Autodesk Inventor part; units mm, degrees
ref_plane "Work Plane1" through (0, 0, 0) normal (0, 0, 1) x (1, 0, 0)
ref_plane "YZ Plane" through (0, 0, 0) normal (1, 0, 0) x (0, 1, 0)
ref_plane "XZ Plane" through (0, 0, 0) normal (0, 1, 0) x (-1, 0, 0)
ref_plane "Work Plane1" through (0, 0, 0) normal (0, 0, 1) x (1, 0, 0)
sketch "Sketch1" plane through (0, 0, 0) normal (0, 0, 1) x (1, 0, 0)
  arc A0 (-0.0454, -1100) -> (0.0454, -1099.9979) centre (-0.0454, -1098) ccw
  line L0 (0.0454, -1099.9979) -> (975.903, -1055.6408)
  arc A1 (975.903, -1055.6408) -> (1100, -925.7749) centre (970, -925.7749) ccw
  line L1 (1100, -174.2251) -> (1100, -925.7749)
  arc A2 (1100, -174.2251) -> (975.903, -44.3592) centre (970, -174.2251) ccw
  line L2 (0.0454, -0.0021) -> (975.903, -44.3592)
  arc A3 (0.0454, -0.0021) -> (-0.0454, 0) centre (-0.0454, -2) ccw
  line L3 (-0.0454, 0) -> (-470, 0)
  arc A4 (-470, 0) -> (-600, -130) centre (-470, -130) ccw
  line L4 (-600, -970) -> (-600, -130)
  arc A5 (-600, -970) -> (-470, -1100) centre (-470, -970) ccw
  line L5 (-0.0454, -1100) -> (-470, -1100)
  point P0 (0, 0)
extrude "Plate1" add sketch "Sketch1" against normal blind 1.5
equation "\"d0\" = Thickness"
equation "\"BendRadius\" = Thickness"
equation "\"BendReliefWidth\" = Thickness"
equation "\"BendReliefDepth\" = 0.5 * Thickness"
equation "\"CornerReliefSize\" = 4 * Thickness"
equation "\"MinimumRemnant\" = 2 * Thickness"
equation "\"TransitionRadius\" = BendRadius"
equation "\"JacobiRadiusSize\" = BendRadius"
equation "\"GapSize\" = Thickness"
properties part number "CARCASA_ALUM_4"
Part model, mm, in its own coordinate system. Round coordinates to 2 decimals unless told otherwise and drop trailing zeros. Loops run counter-clockwise (first coordinate to the right, second up) from the corner with the lowest first, then second, coordinate; pieces in that order, holes last. Notation, with made-up numbers: (54.5, 5.25) -> (63.5, 5.25) arc R23 ccw to (63.5, 31.25) -> close; hole circle Ø11 at (51.5, 35). An arc over 180 degrees is marked (long way). Use a Markdown table: item, result.
1) Cut at C-C, the plane y = -90. List the corners of the cut face in (x, z).
The answers:
| item | result |
|---|---|
| outline | (-593.69, -1.5) -> (1069.03, -1.5) -> (1069.03, 0) -> (-593.69, 0) -> close |
2) Cut at A-A, the plane z = -0.3. List the corners of the cut face in (x, y).
The answers:
| item | result |
|---|---|
| outline | (-600, -970) arc R130 ccw to (-470, -1100) -> (-0.05, -1100) arc R1.93 ccw to (0.05, -1100) -> (975.9, -1055.64) arc R130 ccw to (1100, -925.77) -> (1100, -174.23) arc R130 ccw to (975.9, -44.36) -> (0.05, 0) arc R2.08 ccw to (-0.05, 0) -> (-470, 0) arc R130 ccw to (-600, -130) -> close |
3) Cut at B-B, the plane x = 270.5. List the corners of the cut face in (y, z).
The answers:
| item | result |
|---|---|
| outline | (-1087.7, -1.5) -> (-12.3, -1.5) -> (-12.3, 0) -> (-1087.7, 0) -> close |
4) Probe line 1 (X direction, y = -955, z = -1.3); line 2 (Y direction, x = 97, z = -1); line 3 (Y direction, x = 915.5, z = -0.7). List the from-to ranges inside material, lowest first. Write a range as [from, to].
The answers:
| item | result |
|---|---|
| line 1 | x = [-600, 1096.67] |
| line 2 | y = [-1095.59, -4.41] |
| line 3 | y = [-1058.39, -41.61] |
5) Pull direction X, two halves, no side cores. Call faces 1 (the cylindrical face through (1063.02, -1016.59, -0.74)), 2 (the flat face through (238, -542, -1.5)), 3 (the cylindrical face through (-562.929, -1060.908, -0.74)): pulls with the +X half, pulls with the -X half, needs draft (parallel to the pull), parting line crosses it, or undercut.
The answers:
| item | result |
|---|---|
| face 1 | pulls with the +X half |
| face 2 | needs draft |
| face 3 | pulls with the -X half |
